```python
from build123d import *

# Parameters (mm, degrees)
SKETCH1_R           = 128.5875
BOSS_EXTRUDE1_DEPTH = 2
SKETCH2_R           = 117.475
BOSS_EXTRUDE2_DEPTH = 100
BOSS_EXTRUDE2_TAPER = 30
SKETCH6_R           = 59.739973081
BOSS_EXTRUDE3_DEPTH = 25


with BuildPart() as part:
    # Sketch1 → Boss-Extrude1 (new body)
    with BuildSketch(Plane(origin=(0, 0, 0), x_dir=(1, 0, 0), z_dir=(0, 1, 0))):
        with Locations(Location((0, 0, 0), (0, 0, 270))):
            Circle(SKETCH1_R)
    extrude(amount=BOSS_EXTRUDE1_DEPTH)

    # Sketch2 → Boss-Extrude2 (add)
    with BuildSketch(Plane(origin=(0, 2, 0), x_dir=(1, 0, 0), z_dir=(0, 1, 0))):
        Circle(SKETCH2_R)
    extrude(amount=BOSS_EXTRUDE2_DEPTH, taper=BOSS_EXTRUDE2_TAPER)

    # Sketch6 → Boss-Extrude3 (add)
    with BuildSketch(Plane(origin=(0, 102, 0), x_dir=(1, 0, 0), z_dir=(0, 1, 0))):
        with Locations(Location((0, 0, 0), (0, 0, 270))):
            Circle(SKETCH6_R)
    extrude(amount=BOSS_EXTRUDE3_DEPTH)


solid = part.part
```
Model file for the job. Use its own axes, mm. A direction names the side the tool comes from. Coordinates: 2 decimals unless noted, no trailing zeros. Order: outer loops, then holes, each group sorted by start corner. A loop starts at its lowest first (then second) coordinate and runs counter-clockwise, first axis right, second up. Notation, with made-up numbers: (16, -5.5) - (40, -5.5) arc R21 ccw to (40, -1.5) - close; hole circle Ø7 at (-28.75, 31). An arc over 180 degrees is marked (long way). Return JSON: item names as keys, results as strings. Group by question number.
1) Flat gauge pins, fed straight in: P1, Ø5, axis at x = -39, y = 41, coming from the -Z side; P2, Ø5, axis at x = 70, y = 70, coming from the -Z side; P3, Ø5, axis at y = 19.5, z = -38, coming from the +X side; P4, Ø1.5, axis at x = 40.5, z = 16, coming from the -Y side. Where does each tip first touch, or does it go through?
2) Saw through at B-B, the plane y = 34.5. Write the cut outline in (x, z), plus the area to 3 significant figures.
3) Tool access for faces 1 (the flat face through (2, 0, -2)), 2 (the cylindrical face through (-58.32, 114.32, -12.95)): list every direction of +Z, -Z, +X, -X, +Y, -Y with a clear straight run to the whole face (end or side of a thin tool).
4) Saw through at A-A, the plane x = 0. Write the cut outline in (y, z) (1 decimal).
5) Saw through at C-C, the plane y = 75.5. Write the cut outline in (x, z), plus the area to 3 significant figures.
6) Probe line 1 (Y direction, x = 53, z = -114.5); line 2 (X direction, y = 56, z = 30.5); line 3 (Y direction, x = -114, z = -11.5). List the from-to ranges inside material, lowest first. Write a range as from..to.
Values found:
{
 "1": {"P1": "stops at z = -88.5", "P2": "stops at z = -40.38", "P3": "stops at x = 102.22", "P4": "stops at y = 0"},
 "2": {"outline": "circle Ø197.42 at (0, 0)", "area": "30,600 mm²"},
 "3": {"face 1": "+Z, -Z, +X, -X, -Y", "face 2": "+Y"},
 "4": {"outline": "(0, -128.6) - (2, -128.6) - (2, -117.5) - (102, -59.7) - (127, -59.7) - (127, 59.7) - (102, 59.7) - (2, 117.5) - (2, 128.6) - (0, 128.6) - close"},
 "5": {"outline": "circle Ø150.08 at (0, 0)", "area": "17,700 mm²"},
 "6": {"line 1": "y = 0..2", "line 2": "x = -80.73..80.73", "line 3": "y = 0..7.02"}
}
